from build123d import *

# Parameters (mm, degrees)
F0_R     = 15.126169
F0_W     = 7.62
F0_H     = 4.5212
F1_DEPTH = 7.62
F2_R     = 1.271709
F3_DEPTH = 32.9692
F4_R     = 1.27
F5_DEPTH = 32.766


with BuildPart() as f1:
    # F0 (on Top) → F1 (new body)
    with BuildSketch(Plane.XY):
        Polygon((30.0482, 30.0482), (-30.0482, 30.0482), (-30.0482, 17.6022), (-30.0482, 13.081), (-30.0482, 2.2606), (-30.0482, -2.2606), (-30.0482, -13.081), (-30.0482, -17.6022), (-30.0482, -30.0482), (30.0482, -30.0482), align=None)
        Circle(F0_R, mode=Mode.SUBTRACT)
        with Locations((-33.8582, 15.3416)):
            Rectangle(F0_W, F0_H)
        with Locations((-33.8582, 0)):
            Rectangle(F0_W, F0_H)
        with Locations((-33.8582, -15.3416)):
            Rectangle(F0_W, F0_H)
    extrude(amount=F1_DEPTH)

    # F2 (on Right) → F3 (cut)
    with BuildSketch(Plane.YZ):
        with Locations((26.236491, 3.808291)):
            Circle(F2_R)
    extrude(amount=-F3_DEPTH, mode=Mode.SUBTRACT)

    # F4 (on Right) → F5 (cut)
    with BuildSketch(Plane.YZ):
        with Locations((-26.2382, 3.81)):
            Circle(F4_R)
    extrude(amount=-F5_DEPTH, mode=Mode.SUBTRACT)


solid = f1.part
Input: part model. Units: mm. Frame: model coordinates. A direction names the side the tool comes from. Coordinates: 2 decimals unless noted, no trailing zeros. Loops run counter-clockwise (first coordinate to the right, second up) from the corner with the lowest first, then second, coordinate; pieces in that order, holes last. Notation, with made-up numbers: (-16, 69.5) - (43, 69.5) arc R16 cw to (43, 75.5) - close; hole circle Ø4 at (22, -36). An arc over 180 degrees is marked (long way). Answer in a Markdown table with one row per item. Add a question column.
Item 1: Section query C-C on z = 1.5. Return the cut outline in (x, y).
Item 2: Section query B-B on x = -5.5. Return the cut outline in (y, z), then the cut area to 3 significant figures.
Item 3: Contact query for flat-ended pins moving along their axis: P1, Ø2.5, axis at y = 5.5, z = 5.5, coming from the -X side; P2, Ø4, axis at x = -35.5, z = 4, coming from the +Y side; P3, Ø2.5, axis at x = -34, z = 5, coming from the -Y side. Output: stop coordinate, or through.
Item 4: Section query D-D on x = 5. Return the cut outline in (y, z).
Item 5: Line query: line 1 along Y through (x, z) = (-32, 3); line 2 along Y through (x, z) = (-23, 3.5); line 3 along Y through (x, z) = (0, 2.5). Output: solid intervals per line, ascending. Write a range as [from, to].
Item 6: Mould query, pull axis Y, two halves, no side actions, for faces 1 (the flat face through (-34, 17.602, 4)), 2 (the flat face through (-30.048, 24, 4)), 3 (the flat face through (-30.048, 8, 4)), 4 (the flat face through (-34, 13.081, 4)). Classes: released by +Y, released by -Y, zero draft, split by the parting line, or undercut.
Item 7: Access query for faces 5 (the flat face through (-34, 2.261, 4)), 6 (the cylindrical face through (-14.814, -25.065, 3.324)), 7 (the flat face through (-12, 14, 0)), 8 (the flat face through (-30.048, -24, 4)). Directions: +Z, -Z, +X, -X, +Y, -Y. A direction counts if a zero-diameter tool reaches every point of the face in a straight line with its end or side. Return the directions, or none.
Item 8: Section query A-A on y = 0. Return the cut outline in (x, z), then the cut area to 3 significant figures.
Recorded:
| question | item | result |
|---|---|---|
| 1 | outline | (-37.67, -17.6) - (-30.05, -17.6) - (-30.05, -30.05) - (30.05, -30.05) - (30.05, 30.05) - (-30.05, 30.05) - (-30.05, 17.6) - (-37.67, 17.6) - (-37.67, 13.08) - (-30.05, 13.08) - (-30.05, 2.26) - (-37.67, 2.26) - (-37.67, -2.26) - (-30.05, -2.26) - (-30.05, -13.08) - (-37.67, -13.08) - close; hole circle Ø30.25 at (0, 0) |
| 2 | outline | (-30.05, 0) - (-14.09, 0) - (-14.09, 7.62) - (-30.05, 7.62) - close; (14.09, 0) - (30.05, 0) - (30.05, 7.62) - (14.09, 7.62) - close; hole circle Ø2.54 at (-26.24, 3.81); hole circle Ø2.54 at (26.24, 3.81) |
| 2 | area | 233 mm^2 |
| 3 | P1 | x = -30.05 |
| 3 | P2 | y = 17.6 |
| 3 | P3 | y = -17.6 |
| 4 | outline | (-30.05, 0) - (-14.28, 0) - (-14.28, 7.62) - (-30.05, 7.62) - close; (14.28, 0) - (30.05, 0) - (30.05, 7.62) - (14.28, 7.62) - close |
| 5 | line 1 | [-17.6, -13.08], [-2.26, 2.26], [13.08, 17.6] |
| 5 | line 2 | [-30.05, -27.47], [-25.01, 25], [27.47, 30.05] |
| 5 | line 3 | [-30.05, -15.13], [15.13, 30.05] |
| 6 | face 1 | released by +Y |
| 6 | face 2 | zero draft |
| 6 | face 3 | undercut |
| 6 | face 4 | undercut |
| 7 | face 5 | +Z, -Z, -X |
| 7 | face 6 | -X |
| 7 | face 7 | -Z, +X, -X, +Y, -Y |
| 7 | face 8 | +Z, -Z, -X, -Y |
| 8 | outline | (-37.67, 0) - (-15.13, 0) - (-15.13, 7.62) - (-37.67, 7.62) - close; (15.13, 0) - (30.05, 0) - (30.05, 7.62) - (15.13, 7.62) - close |
| 8 | area | 285 mm^2 |
